Verification items for this drawing (mm, ordinates from the low corner). Coordinates: 2 decimals unless noted, no trailing zeros. Order: outer loops, then holes, each group sorted by start corner. A loop starts at its lowest first (then second) coordinate and runs counter-clockwise, first axis right, second up.
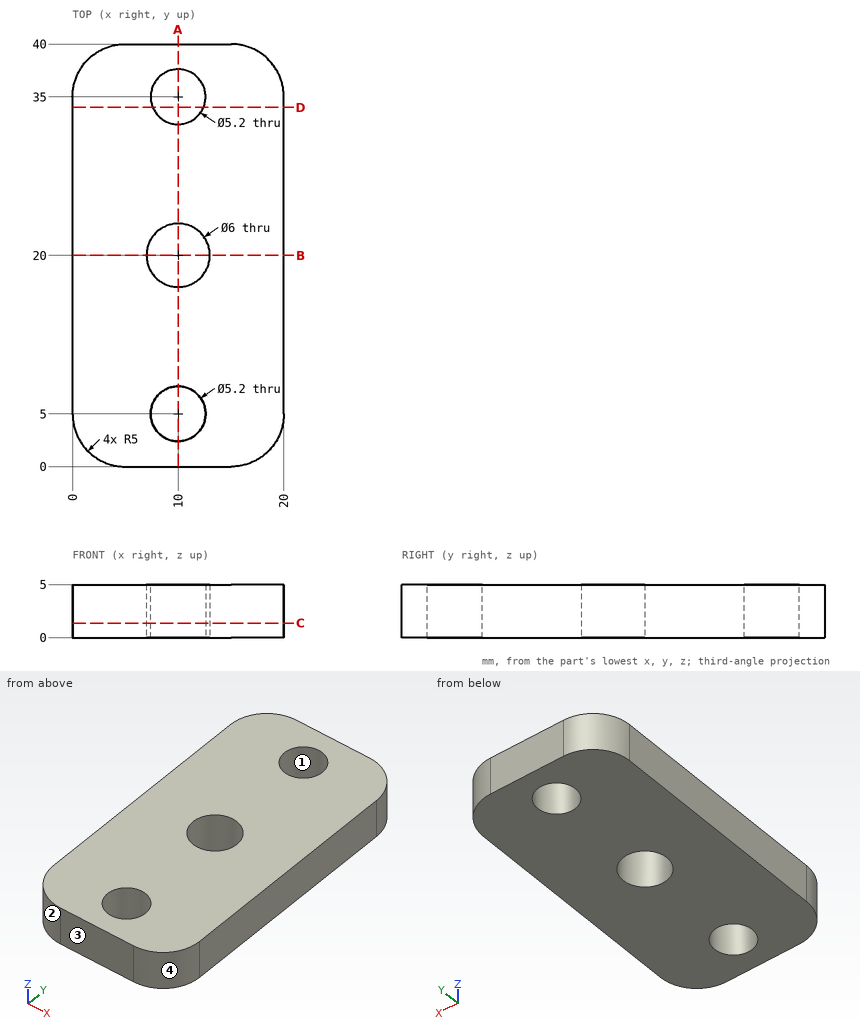
(1) Thickness scan on probe 1 along Y at (x, z) = (10, 1.5); probe 2 along X at (y, z) = (5, 2.8); probe 3 along Y at (x, z) = (15.25, 4.45). Record the ranges inside material, lowest first.
Filled in:
probe 1: y = 0 to 2.4, 7.6 to 17, 23 to 32.4, 37.6 to 40
probe 2: x = 0 to 7.4, 12.6 to 20
probe 3: y = 0.01 to 39.99
(2) Cross-section at C-C (z = 1.35). Enter the section's corners in (x, y), and give its area (3 significant figures).
Filled in:
outline: (0, 5) arc R5 ccw to (5, 0) - (15, 0) arc R5 ccw to (20, 5) - (20, 35) arc R5 ccw to (15, 40) - (5, 40) arc R5 ccw to (0, 35) - close; hole circle Ø6 at (10, 20); hole circle Ø5.2 at (10, 5); hole circle Ø5.2 at (10, 35)
area: 708 mm2
(3) Cross-section at A-A (x = 10). Enter the section's corners in (y, z).
Filled in:
outline: (0, 0) - (2.4, 0) - (2.4, 5) - (0, 5) - close; (7.6, 0) - (17, 0) - (17, 5) - (7.6, 5) - close; (23, 0) - (32.4, 0) - (32.4, 5) - (23, 5) - close; (37.6, 0) - (40, 0) - (40, 5) - (37.6, 5) - close
(4) Cross-section at B-B (y = 20). Enter the section's corners in (x, z), and give its area (3 significant figures).
Filled in:
outline: (0, 0) - (7, 0) - (7, 5) - (0, 5) - close; (13, 0) - (20, 0) - (20, 5) - (13, 5) - close
area: 70.0 mm2
(5) Cross-section at D-D (y = 34). Enter the section's corners in (x, z).
Filled in:
outline: (0, 0) - (7.6, 0) - (7.6, 5) - (0, 5) - close; (12.4, 0) - (20, 0) - (20, 5) - (12.4, 5) - close
(6) Release check for a two-part mould opening along X. For the marked faces 1, 2, 3 and 4 record: +X half, -X half, draft (parallel to the pull), parting line (faces both ways), or undercut.
Filled in:
face 1: undercut
face 2: -X half
face 3: draft
face 4: +X half
(7) Go/stop test with flat-tipped pins: P1, Ø3, axis at x = 10, y = 5, coming from the -Z side; P2, Ø9.5, axis at x = 10, y = 20, coming from the -Z side; P3, Ø3, axis at x = 2.5, z = 4, coming from the +Y side. Record where each tip stops, or that it passes through.
Filled in:
P1: passes through
P2: stops at z = 0
P3: stops at y = 39.9
